Can you work these out from the model? Positions are in its coordinate system, mm. Round coordinates to 2 decimals unless told otherwise and drop trailing zeros. Order: outer loops, then holes, each group sorted by start corner. A loop starts at its lowest first (then second) coordinate and runs counter-clockwise, first axis right, second up. Notation, with made-up numbers: (-23, 54) -> (-14, 54) arc R19 cw to (-14, 70) -> close; hole circle Ø4 at (24.5, 66). An arc over 180 degrees is marked (long way). Use a Markdown table: item, result. Add a question column.
Q1. I'm going to push a flat-ended pin straight in: pin 1 Ø6 at (x, y) = (307, 2.5) entering from -Z. Where does the tip first touch, or does it pass through?
Q2. If we section it at A-A on x = 158: List the corners of the cut face in (y, z) for me, plus the area to 3 significant figures.
Q3. I need wall thicknesses on line 1 along X through (y, z) = (4, 2); line 2 along Y through (x, z) = (109, 0.75); line 3 along Z through (x, y) = (185.5, -2.25). Which ranges of each line are inside material? Lowest first, please. Write a range as [from, to].
Autodesk Inventor part; units mm, degrees
ref_plane "Start Plane" through (0, 0, 0) normal (1, 0, 0) x (0, 1, 0)
ref_plane "XZ Plane" through (0, 0, 0) normal (0, 1, 0) x (-1, 0, 0)
ref_plane "XY Plane" through (0, 0, 0) normal (0, 0, 1) x (1, 0, 0)
sketch "Main Sketch" plane through (0, 0, 0) normal (0, 0, 1) x (1, 0, 0)
  line L0 (0, 0) -> (460, 0)
  line L1 (460, 5) -> (460, 0)
  line L2 (10, 5) -> (460, 5)
  line L3 (0, 0) -> (0, 5)
  line L4 (0, 5) -> (10, 5)
  dimension "d3" = 10
  dimension "d15" = 10
revolve "Revolution1" add sketch "Main Sketch" angle 360 about axis through (0, 0, 0) along (1, 0, 0)
chamfer "Chamfer4" distance 0.595 angle 45 1 edges at (0, -5, 0) measured on face at (3.3333, 4.9353, -0.8021)
chamfer "Chamfer3" distance 0.595 angle 45 1 edges at (460, -5, 0) measured on face at (160, 4.9838, -0.4023)
properties part number "Eje Principal - Interno" material "Aluminum 6061"
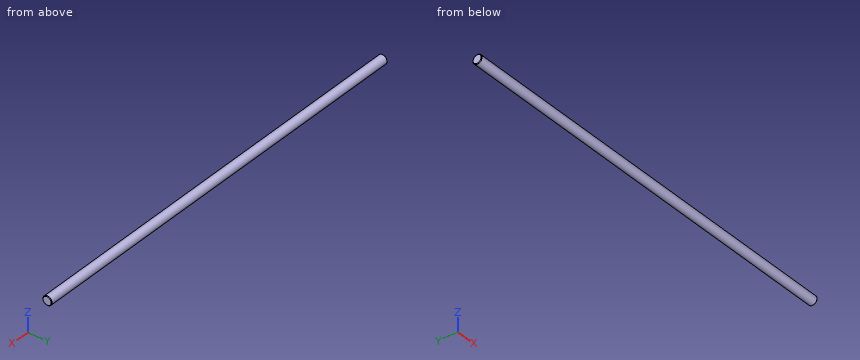
Answer below:
| question | item | result |
|---|---|---|
| 1 | pin 1 | z = -5 |
| 2 | outline | circle Ø10 at (0, 0) |
| 2 | area | 78.5 mm² |
| 3 | line 1 | [0.07, 459.93] |
| 3 | line 2 | [-4.94, 4.94] |
| 3 | line 3 | [-4.47, 4.47] |
